For this review, use the dimensioned drawing (mm, ordinates from the lowest corner) and the shaded views. Coordinates: 2 decimals unless noted, no trailing zeros. Loops run counter-clockwise (first coordinate to the right, second up) from the corner with the lowest first, then second, coordinate; pieces in that order, holes last. Notation, with made-up numbers: (17.5, 83) - (59.5, 83) arc R17 cw to (59.5, 101) - close; hole circle Ø11 at (60, 88.5). An arc over 180 degrees is marked (long way). Answer in a Markdown table with one row per item. Add a question column.
(1) To check wall thickness, follow L1, parallel to Y at x = 31, z = 0.9; L2, parallel to Y at x = 57, z = 2.25; L3, parallel to X at y = 19, z = 2.35. State the ranges of each line that lie inside material, in increasing order. Write a range as [from, to].
(2) We need section A-A, the plane y = 30. Write out the cut boundary in (x, z), plus the area to 3 significant figures.
(3) We need section C-C, the plane x = 61. Write out the cut boundary in (y, z), plus the area to 3 significant figures.
(4) We need section B-B, the plane z = 1.3. Give the number of separate pieces and of enclosed holes in the cut face, plus the area to 3 significant figures.
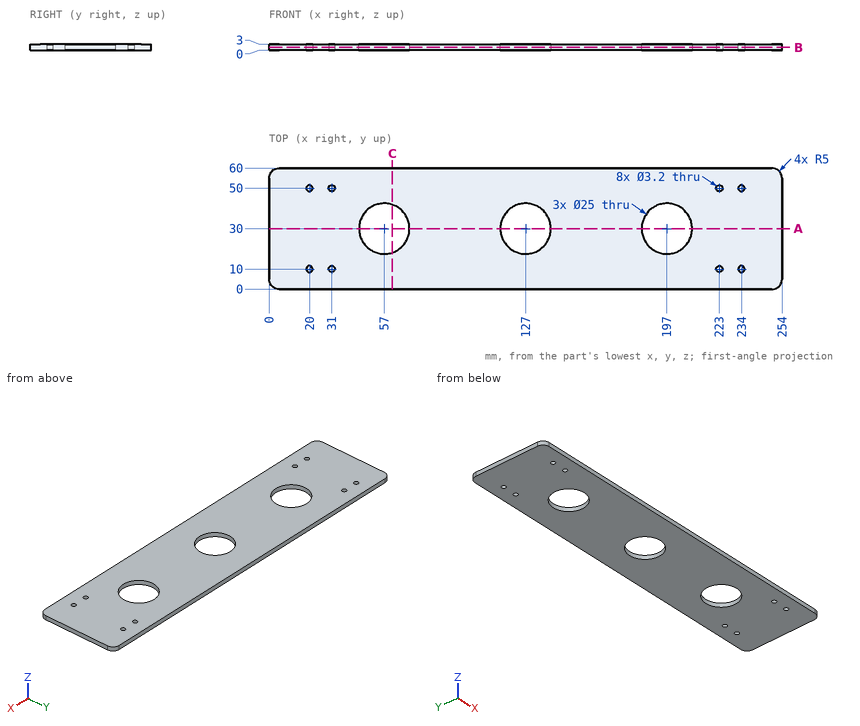
Responses:
| question | item | result |
|---|---|---|
| 1 | L1 | y = [0, 8.4], [11.6, 48.4], [51.6, 60] |
| 1 | L2 | y = [0, 17.5], [42.5, 60] |
| 1 | L3 | x = [0, 51.06], [62.94, 121.06], [132.94, 191.06], [202.94, 254] |
| 2 | outline | (0, 0) - (44.5, 0) - (44.5, 3) - (0, 3) - close; (69.5, 0) - (114.5, 0) - (114.5, 3) - (69.5, 3) - close; (139.5, 0) - (184.5, 0) - (184.5, 3) - (139.5, 3) - close; (209.5, 0) - (254, 0) - (254, 3) - (209.5, 3) - close |
| 2 | area | 537 mm2 |
| 3 | outline | (0, 0) - (18.16, 0) - (18.16, 3) - (0, 3) - close; (41.84, 0) - (60, 0) - (60, 3) - (41.84, 3) - close |
| 3 | area | 109 mm2 |
| 4 | separate pieces | 1 |
| 4 | enclosed holes | 11 |
| 4 | area | 13,700 mm2 |
